Could you check a few things on this model? Use its own coordinates, in mm. Face numbers are marked on the shaded views. A direction names the side the tool comes from. Give positions to 0.01 mm unless a question says otherwise; leave off trailing zeros. Put each result on its own line as item: value.
```python
from build123d import *

# Parameters (mm, degrees)
F0_R      = 68.2625
F1_DEPTH  = 25.4
F2_R      = 38.1
F3_DEPTH  = 101.6
F4_R      = 19.05
F5_DEPTH  = 101.6
F6_R      = 22.225
F7_DEPTH  = 76.2
F8_R      = 5.08
F9_DEPTH  = 25.4
F10_SIZE  = 1.905
F11_DEPTH = 101.6


with BuildPart() as f1:
    # F0 (on Top) → F1 (new body)
    with BuildSketch(Plane.XY):
        Circle(F0_R)
    extrude(amount=F1_DEPTH)

    # F2 (on face) → F3 (join)
    with BuildSketch(Plane(origin=(0, 0, 0), x_dir=(1, 0, 0), z_dir=(0, 0, -1))):
        Circle(F2_R)
    extrude(amount=F3_DEPTH)

    # F4 (on face) → F5 (cut)
    with BuildSketch(Plane.XY.offset(25.4)):
        Circle(F4_R)
    extrude(amount=-F5_DEPTH, mode=Mode.SUBTRACT)

    # F6 (on face) → F7 (cut)
    with BuildSketch(Plane.XY.offset(-76.2)):
        Circle(F6_R)
    extrude(amount=-F7_DEPTH, mode=Mode.SUBTRACT)

    # F8 (on face) → F9 (cut)
    with BuildSketch(Plane.XY.offset(25.4)):
        with Locations((0, 58.42)):
            Circle(F8_R)
        with Locations((-50.5932040891, 29.21)):
            Circle(F8_R)
        with Locations((-50.5932040891, -29.21)):
            Circle(F8_R)
        with Locations((0, -58.42)):
            Circle(F8_R)
        with Locations((50.5932040891, -29.21)):
            Circle(F8_R)
        with Locations((50.5932040891, 29.21)):
            Circle(F8_R)
    extrude(amount=-F9_DEPTH, mode=Mode.SUBTRACT)

    # F10
    f10_edges = [f1.edges().sort_by_distance(p)[0] for p in [
        (-68.2625, 0, 25.4),
        (-68.2625, 0, 0),
    ]]
    chamfer(f10_edges, length=F10_SIZE)

    # F11 (cut): a face of the model
    f11_faces = [f1.faces().sort_by_distance(p)[0] for p in [
        (-37.0223692655, 0, -101.6),
    ]]
    extrude(f11_faces, amount=-F11_DEPTH, mode=Mode.SUBTRACT)


solid = f1.part
```
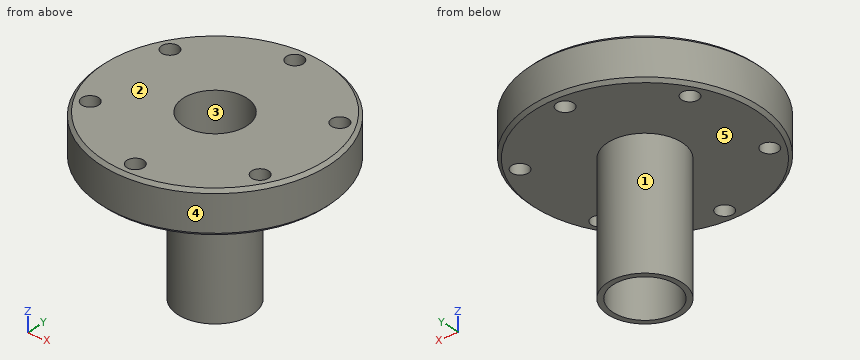
1. For the marked faces 1 and 2, which set-ups out of +Z, -Z, +X, -X, +Y, -Y let a thin tool reach every point of the face, with its end or its side?
Recorded:
face 1: -Z
face 2: +Z, +X, -X, +Y, -Y
2. Thinking about a two-plate mould opening in Y: for the marked faces 3, 4 and 5, which applies, pulls with the +Y half, pulls with the -Y half, needs draft (parallel to the pull), parting line crosses it, or undercut?
Recorded:
face 3: undercut
face 4: parting line crosses it
face 5: needs draft
3. If we section it at B-B (x = 0): Count the separate pieces of the cut face and the enclosed holes in it, then the cut area to 3 significant figures.
Recorded:
separate pieces: 4
enclosed holes: 0
area: 2,460 mm^2
4. I need wall thicknesses on line 1 (Y direction, x = 0, z = 13); line 2 (X direction, y = 29, z = 5); line 3 (Y direction, x = 50, z = 13). Which ranges of each line are inside material? Lowest first, please.
Recorded:
line 1: y = -68.26 to -63.5, -53.34 to -19.05, 19.05 to 53.34, 63.5 to 68.26
line 2: x = -61.8 to -55.67, -45.52 to 45.52, 55.67 to 61.8
line 3: y = -46.47 to -34.26, -24.16 to 24.16, 34.26 to 46.47
5. I'm going to push flat-ended pins straight in: pin 1 (6 mm diameter, centred on x = 20.5, z = -41.5, fed in from -Y); pin 2 (8 mm diameter, centred on y = -16, z = -55.5, fed in from -X); pin 3 (13 mm diameter, centred on x = -50.59, y = -29.21, fed in from +Z); pin 4 (6 mm diameter, centred on y = 18, z = -64.5, fed in from +X). Where does each tip first touch, or does it pass through?
Recorded:
pin 1: stops at y = -13.7
pin 2: stops at x = -18.71
pin 3: stops at z = 25.4
pin 4: stops at x = 16.4
